For this review, use the dimensioned drawing (mm, ordinates from the lowest corner) and the shaded views. Give positions to 0.01 mm unless a question says otherwise; leave off trailing zeros. Loops run counter-clockwise (first coordinate to the right, second up) from the corner with the lowest first, then second, coordinate; pieces in that order, holes last. Notation, with made-up numbers: (-26, 84) -> (-15, 84) arc R29 ccw to (-15, 115) -> close; hole circle Ø6 at (7, -25). An arc over 180 degrees is marked (long way). Write each question's results on one line, items separated by ' | '. Start each with the question number.
Q1. We need section B-B (y = 2.25). Give the number of separate pieces and of enclosed holes in the cut face, plus the area to 3 significant figures.
Q2. Wall thickness on L1, parallel to X at y = 2.4, z = 56; L2, parallel to Z at x = 96, y = 2.65; L3, parallel to X at y = 3.65, z = 20.5: over which ranges is each line inside the solid? List them lowest first. Write a range as [from, to].
Q3. Insertion check: pin 1 Ø1 at (x, y) = (168.5, 3.5) entering from +Z; pin 2 Ø2 at (y, z) = (3, 223.5) entering from +X; pin 3 Ø2 at (x, y) = (123.5, 2.5) entering from -Z. Each pin has a flat end and moves straight along its axis. Give the tip position at first contact, or say it passes through.
Q4. We need section A-A (z = 73). Write out the cut boundary in (x, y).
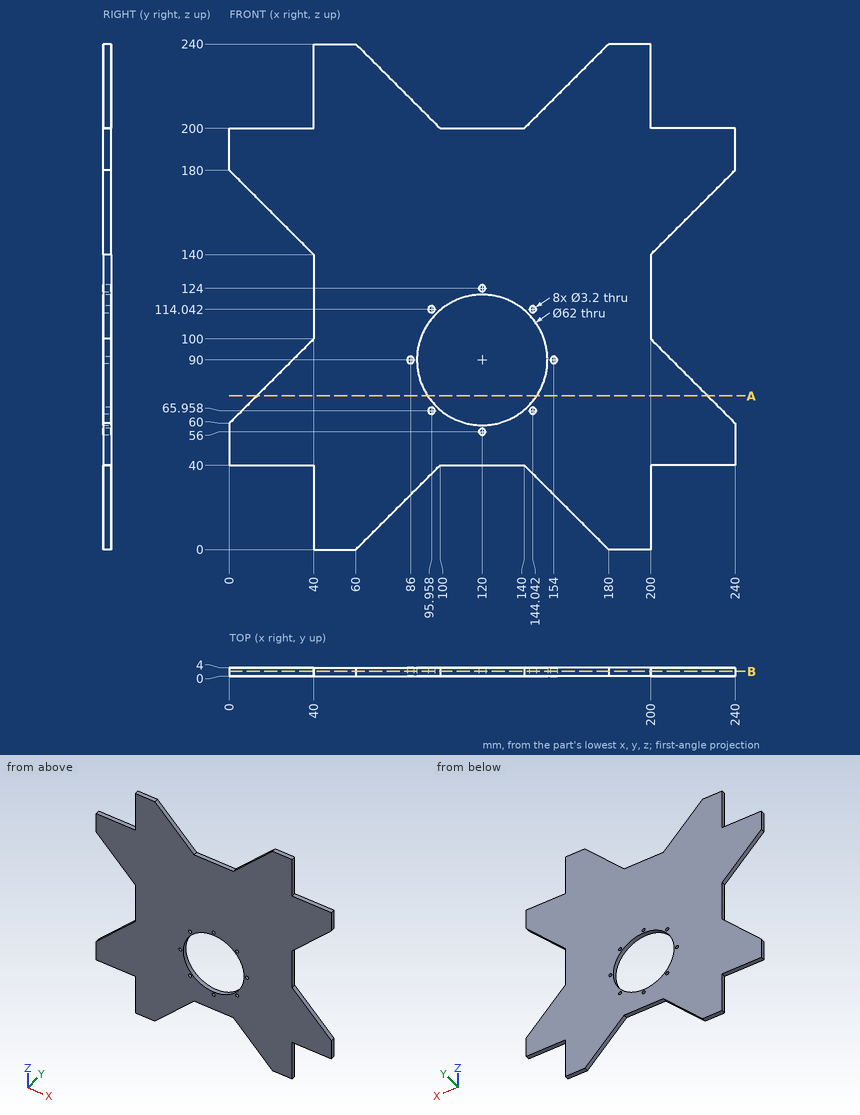
Output:
1) separate pieces: 1 | enclosed holes: 9 | area: 35,300 mm2
2) L1: [0, 118.4], [121.6, 240] | L2: [36, 64.36], [67.56, 70.38], [109.62, 112.44], [115.64, 204] | L3: [40, 80.5], [159.5, 200]
3) pin 1: z = 229 | pin 2: x = 200 | pin 3: z = 40
4) outline: (13, 0) -> (94.08, 0) -> (94.08, 4) -> (13, 4) -> close; (145.92, 0) -> (227, 0) -> (227, 4) -> (145.92, 4) -> close
